Autodesk Fusion 360 part; units mm, degrees
sketch "Sketch1" plane through (0, 0, 0) normal (0, 1, 0) x (1, 0, 0)
  circle A0 centre (0, 0) radius 16.4
  dimension "d1" = 32.8
extrude "Extrude1" add sketch "Sketch1" along normal blind 5
chamfer "Chamfer1" distance 5 distance2 1 1 edges at (-15.2902, 5, 5.9305) measured on face at (3.2266, 5, -3.4774)
sketch "Sketch2" plane through (0, 0, 0) normal (1, 0, 0) x (0, 0, -1)
  line L0 (16.4, 0) -> (17.3, 0)
  line L1 (17.3, 0) -> (17.3, 2)
  line L2 (17.3, 2) -> (16.4, 2)
  line L3 (16.4, 2) -> (16.4, 0)
  line L4 (-16.4, 0) -> (-17.3, 0)
  line L5 (-17.3, 0) -> (-17.3, 2)
  line L6 (-17.3, 2) -> (-16.4, 2)
  line L7 (-16.4, 2) -> (-16.4, 0)
  dimension "d7" = 16.4
  dimension "d8" = 2
  dimension "d9" = 0.9
  dimension "d10" = 16.4
  dimension "d11" = 2
  dimension "d12" = 0.9
revolve "Revolve1" add sketch "Sketch2" angle 4.5 about axis through (0, 1.75, 0) along (0, 1, 0) second angle 4.5
sketch "Sketch3" plane through (0, 0, 0) normal (0, 1, 0) x (1, 0, 0)
  circle A0 centre (0, 0) radius 13.5
  dimension "d15" = 27
extrude "Extrude2" cut sketch "Sketch3" along normal blind 2.78
sketch "Sketch4" plane through (0, 0, 0) normal (0, 0, 1) x (1, 0, 0)
  line L0 (0, 0) -> (16.5, 0)
  line L1 (16.5, 0) -> (16.5, 2)
  line L2 (16.5, 2) -> (0, 2)
  line L3 (0, 2) -> (0, 0)
  dimension "d18" = 16.5
  dimension "d19" = 2
revolve "Revolve2" cut sketch "Sketch4" angle 10 about axis through (0, 1.75, 0) along (0, 1, 0) second angle 10
sketch "Sketch5" plane through (0, 0, 0) normal (1, 0, 0) x (0, 0, -1)
  line L0 (-16.5, 2) -> (-15.5, 2)
  line L1 (-15.5, 2) -> (-15.5, 3)
  line L2 (-15.5, 3) -> (-16.5, 3)
  line L3 (-16.5, 3) -> (-16.5, 2)
  line L4 (16.5, 0) -> (16.5, 2)
  line L5 (16.5, 2) -> (15.5, 2)
  line L6 (15.5, 2) -> (15.5, 3)
  line L7 (15.5, 3) -> (16.5, 3)
  line L8 (16.5, 3) -> (16.5, 2)
  dimension "d24" = 1
  dimension "d25" = 1
  dimension "d28" = 16.5
  dimension "d29" = 2
  dimension "d30" = 1
  dimension "d31" = 1
revolve "Revolve4" cut sketch "Sketch5" angle 4.5 about axis through (0, 1.75, 0) along (0, 1, 0) second angle 4.5 contours L5 L6 L7 L8
revolve "Revolve3" cut sketch "Sketch5" angle 4.5 about axis through (0, 1.75, 0) along (0, 1, 0) second angle 4.5 contours L0 L1 L2 L3
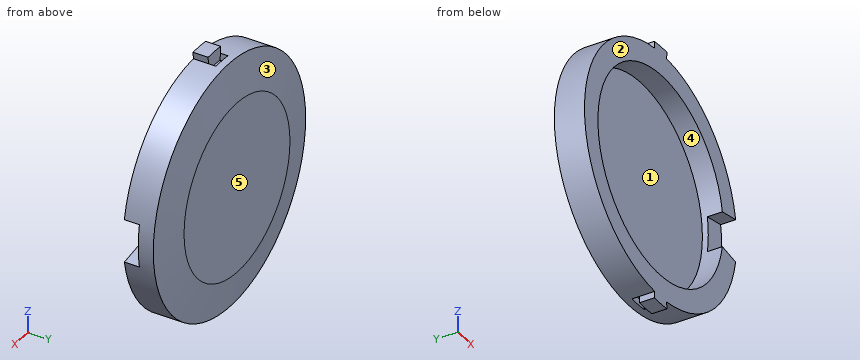
Can you work these out from the model? Positions are in its coordinate system, mm. Face numbers are marked on the shaded views. A direction names the side the tool comes from. Round coordinates to 2 decimals unless told otherwise and drop trailing zeros. Write each loop counter-clockwise with the first axis right and the second up, starting at its lowest first coordinate (ties: lowest second). Pieces come first, ordered by that corner, then holes. Notation, with made-up numbers: (22, 55.5) -> (57, 55.5) arc R20 ccw to (57, 63.5) -> close; hole circle Ø5 at (65.5, 68.5). An arc over 180 degrees is marked (long way). Use one line per item in the form item = value. Start each with the question number.
Q1. Imagine slicing it at D-D (y = 3.55). Please give me the cut outline in (x, z).
Q2. Imagine slicing it at B-B (z = 0). Please give me the cut outline in (x, y).
Q3. Imagine slicing it at A-A (y = 1.45). Please give me the cut outline in (x, z).
Q4. Imagine slicing it at C-C (x = 0). Please give me the cut outline in (y, z), then the cut area to 3 significant figures.
Q5. Which directions (+Z, -Z, +X, -X, +Y, -Y) give clear straight access to the entire face, cutting with the end or side of a thin tool? Please do the marked faces 1 and 2.
Q6. I'm going to push flat-ended pins straight in: P1, Ø0.9, axis at x = 0.5, z = -16.5, coming from the +Y side; P2, Ø1, axis at x = -0.5, z = -16, coming from the -Y side; P3, Ø3, axis at x = -3, y = 3.5, coming from the -Z side; P4, Ø8, axis at x = -5, z = -2, coming from the -Y side. Where does each tip first touch, or does it pass through?
Q7. If I drill on probe 1 along Z at (x, y) = (0, 0.6); probe 2 along Z at (x, y) = (-2.5, 2.4); probe 3 along X at (y, z) = (0.2, 7), over which ranges is the centre line in solid material (lowest first)? Write a range as [from, to].
Q8. We'd pull the mould along Z, two halves only. Please class the marked faces 3, 4 and 5: +Z half, -Z half, draft (parallel to the pull), parting line (faces both ways), or undercut.
Worked out:
q1.outline = circle Ø32.8 at (0, 0)
q2.outline = (-16.4, 0) -> (-13.5, 0) -> (-13.5, 2.78) -> (13.5, 2.78) -> (13.5, 2) -> (16.4, 2) -> (16.4, 4) -> (11.4, 5) -> (-11.4, 5) -> (-16.4, 4) -> close
q3.outline = (-1.36, -17.25) arc R17.3 ccw to (1.36, -17.25) -> (1.29, -16.35) arc R16.4 ccw to (16.15, -2.85) -> (13.29, -2.34) arc R13.5 cw (long way) to (13.29, 2.34) -> (16.15, 2.85) arc R16.4 ccw to (1.29, 16.35) -> (1.36, 17.25) arc R17.3 ccw to (-1.36, 17.25) -> (-1.29, 16.35) arc R16.4 ccw to (-1.29, -16.35) -> close
q4.outline = (0, -17.3) -> (2, -17.3) -> (2, -15.5) -> (3, -15.5) -> (3, -16.4) -> (4, -16.4) -> (5, -11.4) -> (5, 11.4) -> (4, 16.4) -> (3, 16.4) -> (3, 15.5) -> (2, 15.5) -> (2, 17.3) -> (0, 17.3) -> (0, 13.5) -> (2.78, 13.5) -> (2.78, -13.5) -> (0, -13.5) -> close
q4.area = 85.7 mm^2
q5.face_1 = -Y
q5.face_2 = +Z, -Z, +X, -X, -Y
q6.P1 = 4.07
q6.P2 = 0
q6.P3 = -16.33
q6.P4 = 2.78
q7.probe_1 = [-17.3, -13.5], [13.5, 17.3]
q7.probe_2 = [-16.21, -13.27], [13.27, 16.21]
q7.probe_3 = [-14.83, -11.54], [11.54, 14.83]
q8.face_3 = parting line
q8.face_4 = undercut
q8.face_5 = draft
